from build123d import *

# Parameters (mm, degrees)
SKETCH1_W           = 31.75
SKETCH1_H           = 25.4
SKETCH1_R           = 7.1374
SKETCH1_R_2         = 1.2
SKETCH1_R_3         = 1.905
BOSS_EXTRUDE1_DEPTH = 1.5875
BOSS_EXTRUDE3_DEPTH = 1.5875
CUT_EXTRUDE1_DEPTH  = 2.5875
FILLET3_R           = 2.54
FILLET2_R           = 2.286


with BuildPart() as part:
    # Sketch1 → Boss-Extrude1 (new body)
    with BuildSketch(Plane(origin=(0, 0, 0), x_dir=(1, 0, 0), z_dir=(0, 1, 0))):
        Rectangle(SKETCH1_W, SKETCH1_H)
        Circle(SKETCH1_R, mode=Mode.SUBTRACT)
        with Locations((-6.363961031, -6.363961031)):
            Circle(SKETCH1_R_2, mode=Mode.SUBTRACT)
        with Locations((-6.363961031, 6.363961031)):
            Circle(SKETCH1_R_2, mode=Mode.SUBTRACT)
        with Locations((6.363961031, 6.363961031)):
            Circle(SKETCH1_R_2, mode=Mode.SUBTRACT)
        with Locations((6.363961031, -6.363961031)):
            Circle(SKETCH1_R_2, mode=Mode.SUBTRACT)
        with Locations((-12.065, -8.89)):
            Circle(SKETCH1_R_3, mode=Mode.SUBTRACT)
        with Locations((-12.065, 8.89)):
            Circle(SKETCH1_R_3, mode=Mode.SUBTRACT)
        with Locations((12.065, 8.89)):
            Circle(SKETCH1_R_3, mode=Mode.SUBTRACT)
        with Locations((12.065, -8.89)):
            Circle(SKETCH1_R_3, mode=Mode.SUBTRACT)
    extrude(amount=BOSS_EXTRUDE1_DEPTH)

    # Sketch3 → Boss-Extrude3 (add, through all)
    with BuildSketch(Plane(origin=(0, 1.5875, 0), x_dir=(1, 0, 0), z_dir=(0, 1, 0))):
        with BuildLine():
            Line((-3.258830889, 6.35), (3.258830889, 6.35))
            ThreePointArc((3.258830889, 6.35), (0, 7.1374), (-3.258830889, 6.35))
        make_face()
        with BuildLine():
            Line((3.258830889, -6.35), (-3.258830889, -6.35))
            ThreePointArc((-3.258830889, -6.35), (0, -7.1374), (3.258830889, -6.35))
        make_face()
    extrude(amount=-BOSS_EXTRUDE3_DEPTH)

    # Sketch4 → Cut-Extrude1 (cut, through all)
    with BuildSketch(Plane.XZ):
        with BuildLine():
            Line((-15.875, 7.152704943), (-15.875, -7.152704943))
            ThreePointArc((-15.875, -7.152704943), (-12.2174, 0), (-15.875, 7.152704943))
        make_face()
        with BuildLine():
            Line((15.875, -7.152704943), (15.875, 7.152704943))
            ThreePointArc((15.875, 7.152704943), (12.2174, 0), (15.875, -7.152704943))
        make_face()
    extrude(amount=-CUT_EXTRUDE1_DEPTH, mode=Mode.SUBTRACT)

    # Fillet3
    fillet3_edges = [part.edges().sort_by_distance(p)[0] for p in [
        (-15.875, 0.79375, 7.152704943),
        (-15.875, 0.79375, -7.152704943),
        (15.875, 0.79375, 12.7),
        (-15.875, 0.79375, 12.7),
        (15.875, 0.79375, -7.152704943),
        (-15.875, 0.79375, -12.7),
        (15.875, 0.79375, 7.152704943),
        (15.875, 0.79375, -12.7),
    ]]
    fillet(fillet3_edges, radius=FILLET3_R)

    # Fillet2
    fillet2_edges = [part.edges().sort_by_distance(p)[0] for p in [
        (-3.258830889, 0.79375, -6.35),
        (3.258830889, 0.79375, -6.35),
        (3.258830889, 0.79375, 6.35),
        (-3.258830889, 0.79375, 6.35),
    ]]
    fillet(fillet2_edges, radius=FILLET2_R)


solid = part.part
Work out the finished part from the listing and answer in its coordinate system (mm). A direction names the side the tool comes from. Coordinates: 2 decimals unless noted, no trailing zeros. Write each loop counter-clockwise with the first axis right and the second up, starting at its lowest first coordinate (ties: lowest second). Pieces come first, ordered by that corner, then holes. Notation, with made-up numbers: M 12,57.25 L 53,57.25 A15 ccw 53,63.25 Z; hole C 26.25,58.5 d10. An arc over 180 degrees is marked long. Write item = value, one per line.
1. Determine the mould class of faces 4 (the face through (0, 1, 12.7)), 5 (the face through (15.656, 0.805, 7.319)), 6 (the face through (0, 1, 6.35)) for opening direction X: released by +X, released by -X, zero draft, split by the parting line, or undercut.
Solution:
face_4 = zero draft
face_5 = released by +X
face_6 = undercut
2. For faces 1 (the face through (-15.151, 0.805, 11.936)), 2 (the face through (0, 1, -6.35)), 3 (the face through (-15.67, 0.8, 7.35)), determine the directions among +Z, -Z, +X, -X, +Y, -Y from which every point of the face is accessible in a straight line to the end or side of a thin tool.
Solution:
face_1 = +Z, -X, +Y, -Y
face_2 = +Y, -Y
face_3 = -X, +Y, -Y
3. The part is cut by section B-B (x = -3.5). Determine the outline of the cut face in (y, z).
Solution:
outline = M 0,-12.7 L 1.59,-12.7 L 1.59,-6.19 L 0,-6.19 Z; M 0,6.19 L 1.59,6.19 L 1.59,12.7 L 0,12.7 Z
4. The part is cut by section D-D (x = -11.5). Determine the outline of the cut face in (y, z), then the cut area to 3 significant figures.
Solution:
outline = M 0,-12.7 L 1.59,-12.7 L 1.59,-10.71 L 0,-10.71 Z; M 0,-7.07 L 1.59,-7.07 L 1.59,7.07 L 0,7.07 Z; M 0,10.71 L 1.59,10.71 L 1.59,12.7 L 0,12.7 Z
area = 28.8 mm2
5. The part is cut by section A-A (z = 8.89). Determine the outline of the cut face in (x, y) (1 decimal).
Solution:
outline = M -15.9,0 L -14,0 L -14,1.6 L -15.9,1.6 Z; M -10.2,0 L 10.2,0 L 10.2,1.6 L -10.2,1.6 Z; M 14,0 L 15.9,0 L 15.9,1.6 L 14,1.6 Z
6. Straight lines are drawn through the part: line 1 (X direction, y = 0.65, z = -8.89) (3 decimals); line 2 (Z direction, x = -2.5, y = 1.5); line 3 (X direction, y = 1.4, z = 10) (3 decimals). For each, find the intervals that lie inside material, in ascending order. Write a range as from..to.
Solution:
line_1 = -15.875..-13.97, -10.16..10.16, 13.97..15.875
line_2 = -12.7..-6.35, 6.35..12.7
line_3 = -15.875..-13.613, -10.517..10.517, 13.613..15.875
7. The part is cut by section C-C (z = -2.5). Determine the outline of the cut face in (x, y), then the cut area to 3 significant figures.
Solution:
outline = M -12.58,0 L -6.69,0 L -6.69,1.59 L -12.58,1.59 Z; M 6.69,0 L 12.58,0 L 12.58,1.59 L 6.69,1.59 Z
area = 18.7 mm2
